Can you work these out from the model? Positions are in its coordinate system, mm. A direction names the side the tool comes from. Give positions to 0.01 mm unless a question says otherwise; leave off trailing zeros. Write each loop counter-clockwise with the first axis right and the second up, starting at its lowest first coordinate (ties: lowest second). Pieces come first, ordered by that corner, then holes. Notation, with made-up numbers: M 72.5,-23.5 L 98.5,-23.5 A36 cw 98.5,15.5 Z; hole C -17.5,26.5 d8. An arc over 180 degrees is marked long. Write each question's results on one line, items separated by ' | '.
from build123d import *

# Parameters (mm, degrees)
EXTRUDE_1_DEPTH      = 10
EXTRUDE_1_DEPTH_BACK = 8
SKETCH_1_W           = 140.696839698
SKETCH_1_H           = 78.948263704
SKETCH_1_W_2         = 119
SKETCH_1_H_2         = 62
SKETCH_2_W           = 111
SKETCH_2_H           = 62
EXTRUDE_2_DEPTH      = 10
CUT_EXTRUDE_1_DEPTH  = 8
CUT_EXTRUDE_2_DEPTH  = 82.284114443
SKETCH_5_W           = 6
SKETCH_5_H           = 62.061558852
CUT_EXTRUDE_3_DEPTH  = 83.650512768
SKETCH_6_W           = 79.998419849
SKETCH_6_H           = 62.061558852
CUT_EXTRUDE_4_DEPTH  = 4


with BuildPart() as part:
    # 草图1 → 凸台-拉伸1 (new, two sides: drawn at the far end of the back side and taken through both)
    with BuildSketch(Plane.XY.offset(-EXTRUDE_1_DEPTH_BACK)):
        Rectangle(SKETCH_1_W, SKETCH_1_H)
        Rectangle(SKETCH_1_W_2, SKETCH_1_H_2, mode=Mode.SUBTRACT)
    extrude(amount=EXTRUDE_1_DEPTH + EXTRUDE_1_DEPTH_BACK)

    # 草图2 → 凸台-拉伸2 (add)
    with BuildSketch(Plane.XY):
        with Locations((4, 0)):
            Rectangle(SKETCH_2_W, SKETCH_2_H)
    extrude(amount=EXTRUDE_2_DEPTH)

    # 草图3 → 切除-拉伸1 (cut)
    with BuildSketch(Plane.XY.offset(10)):
        Polygon((-51.5, 31), (-26.5, 31), (-26.5, -31.061558852), (-51.5, -31), align=None)
    extrude(amount=-CUT_EXTRUDE_1_DEPTH, mode=Mode.SUBTRACT)

    # 草图4 → 切除-拉伸2 (cut, through all)
    with BuildSketch(Plane.XY.offset(2)):
        Polygon((-51.5, 31), (-47.603613943, 31), (-47.603613943, -31.009594282), (-51.5, -31), align=None)
    extrude(amount=-CUT_EXTRUDE_2_DEPTH, mode=Mode.SUBTRACT)

    # 草图5 → 切除-拉伸3 (cut, through all)
    with BuildSketch(Plane.XY.offset(10)):
        with Locations((56.498419849, -0.030779426)):
            Rectangle(SKETCH_5_W, SKETCH_5_H)
    extrude(amount=-CUT_EXTRUDE_3_DEPTH, mode=Mode.SUBTRACT)

    # 草图6 → 切除-拉伸4 (cut)
    with BuildSketch(Plane.XY.offset(10)):
        with Locations((13.499209925, -0.030779426)):
            Rectangle(SKETCH_6_W, SKETCH_6_H)
    extrude(amount=-CUT_EXTRUDE_4_DEPTH, mode=Mode.SUBTRACT)


solid = part.part
Item 1: For faces 5 (the face through (-26.5, 0, 4)), 6 (the face through (-1, 31, -1)), 7 (the face through (53.498, 0, 4)), 8 (the face through (2, 0, 0)), 9 (the face through (-1, 39.474, 1)), which set-ups out of +Z, -Z, +X, -X, +Y, -Y let a thin tool reach every point of the face, with its end or its side?
Geometry says:
face 5: +Z | face 6: none | face 7: +Z, -Z | face 8: -Z | face 9: +Z, -Z, +X, -X, +Y
Item 2: I want a section at C-C, the plane x = -2.5. Please give me the cut outline in (y, z).
Geometry says:
outline: M -39.47,-8 L -31,-8 L -31,0 L 31,0 L 31,-8 L 39.47,-8 L 39.47,10 L 31,10 L 31,6 L -31.06,6 L -31.06,10 L -39.47,10 Z
Item 3: If I drill on line 1 (X direction, y = -14, z = 3); line 2 (X direction, y = 18.5, z = -2.25); line 3 (Y direction, x = -34, z = -3.25), over which ranges is the centre line in solid material (lowest first)? Write a range as from..to.
Geometry says:
line 1: x = -70.35..-59.5, -26.5..53.5, 59.5..70.35 | line 2: x = -70.35..-59.5, 59.5..70.35 | line 3: y = -39.47..-31, 31..39.47
Item 4: I want a section at A-A, the plane y = 20.5. Give the number of separate pieces and of enclosed holes in the cut face, and give its area (3 significant figures).
Geometry says:
separate pieces: 3 | enclosed holes: 0 | area: 913 mm2
Item 5: I'm going to push flat-ended pins straight in: pin 1 (17 mm diameter, centred on x = -42, y = 3.5, fed in from +Z); pin 2 (3 mm diameter, centred on x = 10, y = -7, fed in from +Z). Where does each tip first touch, or does it pass through?
Geometry says:
pin 1: stops at z = 2 | pin 2: stops at z = 6
Item 6: I want a section at B-B, the plane z = 8.5. Please give me the cut outline in (x, y).
Geometry says:
outline: M -70.35,-39.47 L 70.35,-39.47 L 70.35,39.47 L -70.35,39.47 Z; hole M -59.5,-31 L -51.5,-31 L -26.5,-31.06 L 59.5,-31.06 L 59.5,31 L -59.5,31 Z
Item 7: Thinking about a two-plate mould opening in X: for faces 1 (the face through (2, -31, -4)), 2 (the face through (-1, -39.474, 1)), 3 (the face through (59.5, 0, -4)), 4 (the face through (-70.348, -1, 1)), which applies, +X half, -X half, draft (parallel to the pull), parting line (faces both ways), or undercut?
Geometry says:
face 1: undercut | face 2: draft | face 3: undercut | face 4: -X half
